The model under review builds one solid part; all positions refer to its coordinate system, in mm. A direction names the side the tool comes from. Coordinates: 2 decimals unless noted, no trailing zeros. Loops run counter-clockwise (first coordinate to the right, second up) from the corner with the lowest first, then second, coordinate; pieces in that order, holes last. Notation, with made-up numbers: (75, 54) - (107, 54) arc R21 cw to (107, 90) - close; hole circle Ø5 at (81.25, 16). An arc over 180 degrees is marked (long way). Use a Markdown table: item, result. Add a question column.
1) To check wall thickness, follow L1, parallel to Z at x = 2.5, y = 4.75 (3 decimals); L2, parallel to Z at x = 14, y = 3.5; L3, parallel to X at y = 4, z = -72. State the ranges of each line that lie inside material, in increasing order. Write a range as [from, to].
2) Add section B-B, the plane x = -14.5. Give the boundary of the cut face in (y, z).
3) Add section D-D, the plane x = 35. Give the boundary of the cut face in (y, z), and give its area (3 significant figures).
4) For faces 4 (the flat face through (2, 6.35, 54)), 5 (the flat face through (-1, 3.25, -1)), 6 (the flat face through (-90.442, 3.219, -51.772)), list the 3-axis set-ups (+Z, -Z, +X, -X, +Y, -Y) from which the entire face can be reached by the end or side of a thin tool; tool diameter is ignored.
5) The part is to be moulded in two halves that separate along X. For faces 1 (the cylindrical face through (5.5, 3.13, -124.88)), 2 (the flat face through (2, 0, -2)), 3 (the flat face through (-101.21, 3.22, -26.68)), say which applies: pulls with the +X half, pulls with the -X half, needs draft (parallel to the pull), parting line crosses it, or undercut.
6) Add section C-C, the plane z = 0. Give the boundary of the cut face in (x, y), and give its area (3 significant figures).
7) Clearance check with flat-ended pins moving along their axes: pin 1 (0.9 mm diameter, centred on x = 17.5, y = 4.5, fed in from -Z); pin 2 (0.9 mm diameter, centred on y = 5.5, z = -14, fed in from -X); pin 3 (1.6 mm diameter, centred on y = 4, z = -15, fed in from +X). State where each tip first meets the part, or that it passes through.
8) Add section A-A, the plane y = 4.25. Give the boundary of the cut face in (x, z), and give its area (3 significant figures).
```python
from build123d import *

# Parameters (mm, degrees)
SKETCH1_R           = 125
BOSS_EXTRUDE1_DEPTH = 6.35
SKETCH3_W           = 55
SKETCH3_H           = 6.35
CUT_EXTRUDE1_DEPTH  = 177.890707783
SKETCH4_W           = 106.5
SKETCH4_H           = 106.5
CUT_EXTRUDE2_DEPTH  = 3.1


with BuildPart() as part:
    # Sketch1 → Boss-Extrude1 (new body)
    with BuildSketch(Plane(origin=(0, 0, 0), x_dir=(1, 0, 0), z_dir=(0, 1, 0))):
        with Locations(Location((0, 0, 0), (0, 0, 270))):
            Circle(SKETCH1_R)
    extrude(amount=BOSS_EXTRUDE1_DEPTH)

    # Sketch3 → Cut-Extrude1 (cut, through all)
    with BuildSketch(Plane(origin=(0, 6.35, 0), x_dir=(1, 0, 0), z_dir=(0, 1, 0))):
        Polygon((-98.500369343, 25.11494995), (-103.999630657, 28.28994995), (-76.499630657, 75.921347158), (-71.000369343, 72.746347158), align=None)
        Polygon((71.000369343, 72.746347158), (98.500369343, 25.11494995), (103.999630657, 28.28994995), (76.499630657, 75.921347158), align=None)
        with Locations((0, -101.036297108)):
            Rectangle(SKETCH3_W, SKETCH3_H)
    extrude(amount=-CUT_EXTRUDE1_DEPTH, mode=Mode.SUBTRACT)

    # Sketch4 → Cut-Extrude2 (cut)
    with BuildSketch(Plane(origin=(0, 6.35, 0), x_dir=(1, 0, 0), z_dir=(0, 1, 0))):
        Rectangle(SKETCH4_W, SKETCH4_H)
    extrude(amount=-CUT_EXTRUDE2_DEPTH, mode=Mode.SUBTRACT)


solid = part.part
```
From the geometry:
| question | item | result |
|---|---|---|
| 1 | L1 | z = [-124.975, -53.25], [53.25, 97.861], [104.211, 124.975] |
| 1 | L2 | z = [-124.21, -53.25], [53.25, 97.86], [104.21, 124.21] |
| 1 | L3 | x = [-102.18, -78.76], [-71.43, 71.43], [78.76, 102.18] |
| 2 | outline | (0, -124.16) - (6.35, -124.16) - (6.35, -53.25) - (3.25, -53.25) - (3.25, 53.25) - (6.35, 53.25) - (6.35, 97.86) - (0, 97.86) - close; (0, 104.21) - (6.35, 104.21) - (6.35, 124.16) - (0, 124.16) - close |
| 3 | outline | (0, -120) - (6.35, -120) - (6.35, -53.25) - (3.25, -53.25) - (3.25, 53.25) - (6.35, 53.25) - (6.35, 120) - (0, 120) - close |
| 3 | area | 1,190 mm^2 |
| 4 | face 4 | +Z, -Z, +X, -X, +Y |
| 4 | face 5 | +Y |
| 4 | face 6 | +Y, -Y |
| 5 | face 1 | parting line crosses it |
| 5 | face 2 | needs draft |
| 5 | face 3 | undercut |
| 6 | outline | (-125, 0) - (125, 0) - (125, 6.35) - (53.25, 6.35) - (53.25, 3.25) - (-53.25, 3.25) - (-53.25, 6.35) - (-125, 6.35) - close |
| 6 | area | 1,260 mm^2 |
| 7 | pin 1 | stops at z = -123.83 |
| 7 | pin 2 | stops at x = -124.26 |
| 7 | pin 3 | stops at x = 124.19 |
| 8 | outline | circle Ø250 at (0, 0); hole (-104, -28.29) - (-76.5, -75.92) - (-71, -72.75) - (-98.5, -25.11) - close; hole (-53.25, -53.25) - (53.25, -53.25) - (53.25, 53.25) - (-53.25, 53.25) - close; hole (-27.5, 97.86) - (27.5, 97.86) - (27.5, 104.21) - (-27.5, 104.21) - close; hole (71, -72.75) - (76.5, -75.92) - (104, -28.29) - (98.5, -25.11) - close |
| 8 | area | 36,700 mm^2 |
